Model file for the job. Use its own axes, mm. Round coordinates to 2 decimals unless told otherwise and drop trailing zeros. Order: outer loops, then holes, each group sorted by start corner. A loop starts at its lowest first (then second) coordinate and runs counter-clockwise, first axis right, second up. Notation, with made-up numbers: (49.25, -0.75) -> (58.25, -0.75) arc R20 ccw to (58.25, 38.25) -> close; hole circle Ø7 at (17.25, 46.5). An arc over 180 degrees is marked (long way). Answer as CSV lines item,"result".
Autodesk Inventor part; units mm, degrees
ref_plane "YZ Plane" through (0, 0, 0) normal (1, 0, 0) x (0, 1, 0)
ref_plane "XZ Plane" through (0, 0, 0) normal (0, 1, 0) x (-1, 0, 0)
ref_plane "XY Plane" through (0, 0, 0) normal (0, 0, 1) x (1, 0, 0)
sketch "Sketch1" plane through (0, 0, 0) normal (0, 0, 1) x (1, 0, 0)
  circle A0 centre (0, -12) radius 1.5
  circle A1 centre (0, 12) radius 1.5
  line L0 (3.8971, -14.25) -> (9.0933, -5.25)
  arc A2 (9.0933, -5.25) -> (9.0933, 5.25) centre (0, 0) ccw
  line L1 (9.0933, 5.25) -> (3.8971, 14.25)
  arc A3 (3.8971, 14.25) -> (-3.8971, 14.25) centre (0, 12) ccw
  line L2 (-3.8971, 14.25) -> (-9.0933, 5.25)
  arc A4 (-9.0933, 5.25) -> (-9.0933, -5.25) centre (0, 0) ccw
  line L3 (-9.0933, -5.25) -> (-3.8971, -14.25)
  arc A5 (-3.8971, -14.25) -> (3.8971, -14.25) centre (0, -12) ccw
extrude "Extrusion1" add sketch "Sketch1" along normal blind 6
properties part number "shaftPlug"
Q1. Saw through at B-B (z = 1.15). Write the cut outline in (x, y).
Checks:
outline,"(-9.09, -5.25) -> (-3.9, -14.25) arc R4.5 ccw to (3.9, -14.25) -> (9.09, -5.25) arc R10.5 ccw to (9.09, 5.25) -> (3.9, 14.25) arc R4.5 ccw to (-3.9, 14.25) -> (-9.09, 5.25) arc R10.5 ccw to start; hole circle Ø3 at (0, -12); hole circle Ø3 at (0, 12)"
Q2. Saw through at A-A (x = 0). Write the cut outline in (y, z), plus the area to 3 significant figures.
Checks:
outline,"(-16.5, 0) -> (-13.5, 0) -> (-13.5, 6) -> (-16.5, 6) -> close; (-10.5, 0) -> (10.5, 0) -> (10.5, 6) -> (-10.5, 6) -> close; (13.5, 0) -> (16.5, 0) -> (16.5, 6) -> (13.5, 6) -> close"
area,"162 mm²"
Q3. Mould opens along Y. For faces 1 (the cylindrical face through (-0.325, -10.536, 2.958)), 2 (the flat face through (-6.53, -9.69, 2.96)), 3 (the cylindrical face through (-10.5, -0.1, 3)) say: +Y half, -Y half, draft (parallel to the pull), parting line (faces both ways), or undercut.
Checks:
face 1,"undercut"
face 2,"-Y half"
face 3,"parting line"
Q4. Saw through at C-C (y = -12). Write the cut outline in (x, z).
Checks:
outline,"(-5.2, 0) -> (-1.5, 0) -> (-1.5, 6) -> (-5.2, 6) -> close; (1.5, 0) -> (5.2, 0) -> (5.2, 6) -> (1.5, 6) -> close"
Q5. Flat gauge pins, fed straight in: pin 1 (2 mm diameter, centred on y = -4.5, z = 1.5, fed in from -X); pin 2 (3 mm diameter, centred on x = -3.5, z = 3.5, fed in from -Y); pin 3 (2 mm diameter, centred on y = 5.5, z = 2.5, fed in from -X). Where does each tip first touch, or does it go through?
Checks:
pin 1,"x = -9.9"
pin 2,"y = -16.03"
pin 3,"x = -9.49"
Q6. Saw through at D-D (x = 4.75). Write the cut outline in (y, z), plus the area to 3 significant figures.
Checks:
outline,"(-12.77, 0) -> (12.77, 0) -> (12.77, 6) -> (-12.77, 6) -> close"
area,"153 mm²"
Q7. Wall check: L1, parallel to X at y = -11.5, z = 1.85; L2, parallel to Y at x = -6, z = 0.35; L3, parallel to Y at x = -6.5, z = 0.9. Give the ranges that are in metal, low to high. Write a range as [from, to].
Checks:
L1,"[-5.48, -1.41], [1.41, 5.48]"
L2,"[-10.61, 10.61]"
L3,"[-9.74, 9.74]"
